from build123d import *

# Parameters (mm, degrees)
SKETCH1_W           = 44.45
SKETCH1_H           = 50.8
SKETCH1_R           = 2
SKETCH1_R_2         = 4
BOSS_EXTRUDE1_DEPTH = 3.175
SKETCH3_W           = 44.45
SKETCH3_H           = 3.175
BOSS_EXTRUDE2_DEPTH = 76.2
SKETCH6_W           = 3.175
SKETCH6_H           = 76.2
BOSS_EXTRUDE3_DEPTH = 47.625
CHAMFER1_SIZE       = 44.45
CHAMFER1_SIZE2      = 76.2
SKETCH8_R           = 2.75
CUT_EXTRUDE1_DEPTH  = 96.197068626


with BuildPart() as part:
    # Sketch1 → Boss-Extrude1 (new body)
    with BuildSketch(Plane.XY):
        Rectangle(SKETCH1_W, SKETCH1_H)
        with Locations((0, 8.5)):
            Circle(SKETCH1_R, mode=Mode.SUBTRACT)
        with Locations(Location((0, -8.5, 0), (0, 0, 180))):
            Circle(SKETCH1_R, mode=Mode.SUBTRACT)
        Circle(SKETCH1_R_2, mode=Mode.SUBTRACT)
    extrude(amount=BOSS_EXTRUDE1_DEPTH)

    # Sketch3 → Boss-Extrude2 (add)
    with BuildSketch(Plane.XY.offset(3.175)):
        with Locations((0, -23.8125)):
            Rectangle(SKETCH3_W, SKETCH3_H)
    extrude(amount=BOSS_EXTRUDE2_DEPTH)

    # Sketch6 → Boss-Extrude3 (add)
    with BuildSketch(Plane(origin=(0, -22.225, 0), x_dir=(1, 0, 0), z_dir=(0, 1, 0))):
        with Locations((20.6375, -41.275)):
            Rectangle(SKETCH6_W, SKETCH6_H)
        with Locations((-20.6375, -41.275)):
            Rectangle(SKETCH6_W, SKETCH6_H)
    extrude(amount=BOSS_EXTRUDE3_DEPTH)

    # Chamfer1
    chamfer1_edges = [part.edges().sort_by_distance(p)[0] for p in [
        (-20.6375, 25.4, 79.375),
        (20.6375, 25.4, 79.375),
    ]]
    chamfer1_side = [part.faces().sort_by_distance(p)[0] for p in [
        (0, -24.724985741, 79.375),
    ]]
    chamfer(chamfer1_edges, length=CHAMFER1_SIZE, length2=CHAMFER1_SIZE2, reference=chamfer1_side[0])

    # Sketch8 → Cut-Extrude1 (cut, through all)
    with BuildSketch(Plane(origin=(0, -22.225, 0), x_dir=(1, 0, 0), z_dir=(0, 1, 0))):
        with Locations(Location((-7.9375, -15.875, 0), (0, 0, 270))):
            Circle(SKETCH8_R)
        with Locations(Location((7.9375, -15.875, 0), (0, 0, 270))):
            Circle(SKETCH8_R)
        with Locations(Location((7.9375, -66.675, 0), (0, 0, 270))):
            Circle(SKETCH8_R)
        with Locations(Location((-7.9375, -66.675, 0), (0, 0, 270))):
            Circle(SKETCH8_R)
    extrude(amount=-CUT_EXTRUDE1_DEPTH, mode=Mode.SUBTRACT)


solid = part.part
Source: CAD feature listing. Evaluate the final solid. Frame: model axes, mm. A direction names the side the tool comes from. Coordinates: 2 decimals unless noted, no trailing zeros. Loops run counter-clockwise (first coordinate to the right, second up) from the corner with the lowest first, then second, coordinate; pieces in that order, holes last. Notation, with made-up numbers: (54, 46.5) -> (80, 46.5) arc R23 ccw to (80, 72.5) -> close; hole circle Ø3 at (-23.75, 89). An arc over 180 degrees is marked (long way). Answer in a Markdown table with one row per item. Add a question column.
Q1. Section D-D on x = -18. Return the cut outline in (y, z) (3 decimals), and give its area (3 significant figures).
Q2. Section B-B on y = 0. Return the cut outline in (x, z) (3 decimals), and give its area (3 significant figures).
Q3. Section A-A on x = 0. Return the cut outline in (y, z) (3 decimals).
Q4. Section C-C on z = 14. Return the cut outline in (x, y) (3 decimals), and give its area (3 significant figures).
Q5. Pull-direction query (Y, two-part tool) for faces 1 (the face through (0, -22.225, 41)), 2 (the face through (-0.867, -3.905, 1.565)), 3 (the face through (0, -25.4, 39)), 4 (the face through (22.225, -6, 31)); classes: pulls with the +Y half, pulls with the -Y half, needs draft (parallel to the pull), parting line crosses it, or undercut.
Q6. Reachability of faces 5 (the face through (19.05, -4, 33)), 6 (the face through (0, 25.4, 2)) from +Z, -Z, +X, -X, +Y, -Y: full face, straight path, thin tool, end or side. Return the list, or none.
Q7. Ray query, line 1 along Y through (x, z) = (0, 2); line 2 along X through (y, z) = (-11.5, 55) (3 decimals). Return the intervals inside material, ascending.
Q8. Contact query for flat-ended pins moving along their axis: pin 1 Ø19 at (x, z) = (1.5, 43) entering from +Y (3 decimals); pin 2 Ø10.5 at (x, y) = (0, 0) entering from +Z (3 decimals); pin 3 Ø10 at (x, z) = (14.5, 44.5) entering from +Y. Output: stop coordinate, or through.
Computed values:
| question | item | result |
|---|---|---|
| 1 | outline | (-25.4, 0) -> (25.4, 0) -> (25.4, 3.175) -> (-22.225, 3.175) -> (-22.225, 79.375) -> (-25.4, 79.375) -> close |
| 1 | area | 403 mm^2 |
| 2 | outline | (-22.225, 0) -> (-4, 0) -> (-4, 3.175) -> (-19.05, 3.175) -> (-19.05, 46.718) -> (-22.225, 46.718) -> close; (4, 0) -> (22.225, 0) -> (22.225, 46.718) -> (19.05, 46.718) -> (19.05, 3.175) -> (4, 3.175) -> close |
| 2 | area | 392 mm^2 |
| 3 | outline | (-25.4, 0) -> (-10.5, 0) -> (-10.5, 3.175) -> (-22.225, 3.175) -> (-22.225, 79.375) -> (-25.4, 79.375) -> close; (-6.5, 0) -> (-4, 0) -> (-4, 3.175) -> (-6.5, 3.175) -> close; (4, 0) -> (6.5, 0) -> (6.5, 3.175) -> (4, 3.175) -> close; (10.5, 0) -> (25.4, 0) -> (25.4, 3.175) -> (10.5, 3.175) -> close |
| 4 | outline | (-22.225, -25.4) -> (-9.949, -25.4) -> (-9.949, -22.225) -> (-19.05, -22.225) -> (-19.05, 19.085) -> (-22.225, 19.085) -> close; (-5.926, -25.4) -> (5.926, -25.4) -> (5.926, -22.225) -> (-5.926, -22.225) -> close; (9.949, -25.4) -> (22.225, -25.4) -> (22.225, 19.085) -> (19.05, 19.085) -> (19.05, -22.225) -> (9.949, -22.225) -> close |
| 4 | area | 378 mm^2 |
| 5 | face 1 | pulls with the +Y half |
| 5 | face 2 | undercut |
| 5 | face 3 | pulls with the -Y half |
| 5 | face 4 | needs draft |
| 6 | face 5 | +Z, +Y |
| 6 | face 6 | +Z, -Z, +X, -X, +Y |
| 7 | line 1 | y = -25.4 to -10.5, -6.5 to -4, 4 to 6.5, 10.5 to 25.4 |
| 7 | line 2 | x = -22.225 to -19.05, 19.05 to 22.225 |
| 8 | pin 1 | stops at y = -22.225 |
| 8 | pin 2 | stops at z = 3.175 |
| 8 | pin 3 | stops at y = 2.5 |
